Source: three-view drawing plus pictorial views. Frame: mm from the lowest corner of the part. A direction names the side the tool comes from. Give positions to 0.01 mm unless a question says otherwise; leave off trailing zeros. Loops run counter-clockwise (first coordinate to the right, second up) from the corner with the lowest first, then second, coordinate; pieces in that order, holes last.
1. Section C-C, the plane z = 5.5. Output: boundary loops of the cut face in (x, y) (3 decimals).
2. Material intervals for line 1 along Y through (x, z) = (2.85, 5.5); line 2 along X through (y, z) = (40.45, 7.25); line 3 along X through (y, z) = (22.5, 2.25) (3 decimals), sorted ascending.
3. Section A-A, the plane x = 2.85. Output: boundary loops of the cut face in (y, z), then the cut area to 3 significant figures.
4. Section B-B, the plane y = 40.45. Output: boundary loops of the cut face in (x, z), then the cut area to 3 significant figures.
5. Draft query along X for the marked faces 1, 2 and 3. Return one class per face: +X half, -X half, draft (parallel to the pull), parting line (faces both ways), or undercut.
6. Section D-D, the plane y = 29. Output: boundary loops of the cut face in (x, z) (3 decimals).
7. Access query for the marked faces 4, 5 and 6. Directions: +Z, -Z, +X, -X, +Y, -Y. A direction counts if a zero-diameter tool reaches every point of the face in a straight line with its end or side. Return the directions, or none.
8. First-contact query: P1, Ø4.5, axis at y = 19.5, z = 5, coming from the +X side (3 decimals); P2, Ø4.5, axis at x = 24, z = 6.5, coming from the +Y side (3 decimals); P3, Ø1, axis at x = 35.5, z = 7.5, coming from the -Y side (3 decimals); P4, Ø2, axis at x = 60.45, y = 2.85, coming from the +Z side. Flat tips, straight axial feed; report the tip coordinate or a pass-through.
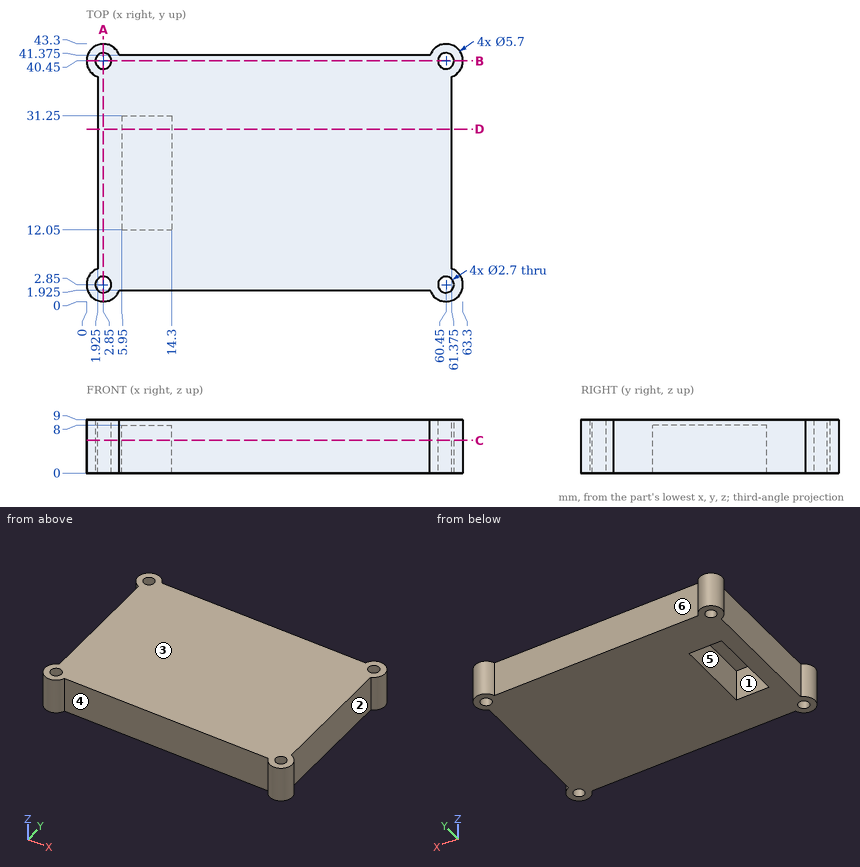
Answers below:
1. outline: (1.925, 5.546) arc R2.85 ccw (long way) to (5.546, 1.925) - (57.754, 1.925) arc R2.85 ccw (long way) to (61.375, 5.546) - (61.375, 37.754) arc R2.85 ccw (long way) to (57.754, 41.375) - (5.546, 41.375) arc R2.85 ccw (long way) to (1.925, 37.754) - close; hole circle Ø2.7 at (2.85, 2.85); hole circle Ø2.7 at (2.85, 40.45); hole (5.95, 12.05) - (14.3, 12.05) - (14.3, 31.25) - (5.95, 31.25) - close; hole circle Ø2.7 at (60.45, 2.85); hole circle Ø2.7 at (60.45, 40.45)
2. line 1: y = 0 to 1.5, 4.2 to 39.1, 41.8 to 43.3
2. line 2: x = 0 to 1.5, 4.2 to 59.1, 61.8 to 63.3
2. line 3: x = 1.925 to 5.95, 14.3 to 61.375
3. outline: (0, 0) - (1.5, 0) - (1.5, 9) - (0, 9) - close; (4.2, 0) - (39.1, 0) - (39.1, 9) - (4.2, 9) - close; (41.8, 0) - (43.3, 0) - (43.3, 9) - (41.8, 9) - close
3. area: 341 mm2
4. outline: (0, 0) - (1.5, 0) - (1.5, 9) - (0, 9) - close; (4.2, 0) - (59.1, 0) - (59.1, 9) - (4.2, 9) - close; (61.8, 0) - (63.3, 0) - (63.3, 9) - (61.8, 9) - close
4. area: 521 mm2
5. face 1: undercut
5. face 2: +X half
5. face 3: draft
6. outline: (1.925, 0) - (5.95, 0) - (5.95, 8) - (14.3, 8) - (14.3, 0) - (61.375, 0) - (61.375, 9) - (1.925, 9) - close
7. face 4: +Z, -Z, -Y
7. face 5: -Z
7. face 6: +Z, -Z, +Y
8. P1: stops at x = 61.375
8. P2: stops at y = 41.375
8. P3: stops at y = 1.925
8. P4: passes through
